Here's how the part is built. I have some questions about the finished solid (model axes, mm). Face numbers are marked on the shaded views. A direction names the side the tool comes from. Coordinates: 2 decimals unless noted, no trailing zeros. Write each loop counter-clockwise with the first axis right and the second up, starting at its lowest first coordinate (ties: lowest second). Pieces come first, ordered by that corner, then holes. Notation, with made-up numbers: (18.5, 41.5) -> (67.5, 41.5) arc R17 cw to (67.5, 73.5) -> close; hole circle Ø4 at (-31, -22). An arc over 180 degrees is marked (long way). Use CSV: the item, a comma, the result in double quotes. Start each with the question number.
```python
from build123d import *

# Parameters (mm, degrees)
SKETCH1_W           = 70
SKETCH1_H           = 170
SKETCH1_W_2         = 40
SKETCH1_H_2         = 140
BOSS_EXTRUDE1_DEPTH = 20


# Read off the part's stored shape, not the designer's step: Hole1
with BuildPart() as part:
    # Sketch1 → Boss-Extrude1 (new body)
    with BuildSketch(Plane(origin=(0, 0, 0), x_dir=(0, 0, -1), z_dir=(1, 0, 0))):
        Rectangle(SKETCH1_W, SKETCH1_H)
        Rectangle(SKETCH1_W_2, SKETCH1_H_2, mode=Mode.SUBTRACT)
    extrude(amount=BOSS_EXTRUDE1_DEPTH)

    # Hole1 outline → Hole1 (revolve, cut)
    with BuildSketch(Plane(origin=(10.287047222, -0.784426919, 0), x_dir=(1, 0, 0), z_dir=(0, -1, 0))):
        Polygon((0, 20), (2.555546136, 20), (2.031734593, 35), (0, 35), align=None)
        Polygon((3.952376915, -20), (0, -20), (0, -35), (4.476188458, -35), align=None)
    revolve(axis=Axis((10.287047222, -0.784426919, 0), (0, 0, 1)), mode=Mode.SUBTRACT)


solid = part.part
```
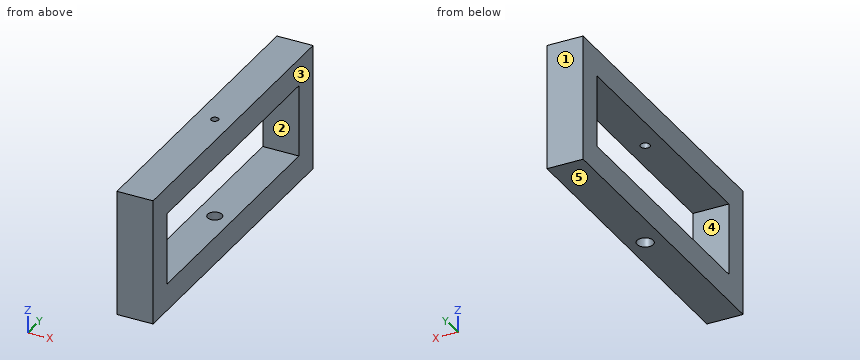
Item 1: If I drill on line 1 along Y through (x, z) = (16, 14); line 2 along Z through (x, y) = (7.5, 59.5); line 3 along Y through (x, z) = (10.75, -28), over which ranges is the centre line in solid material (lowest first)?
Item 2: Thinking about a two-plate mould opening in Y: for the marked faces 1, 2 and 3, which applies, +Y half, -Y half, draft (parallel to the pull), parting line (faces both ways), or undercut?
Item 3: I want a section at A-A on y = -26. Please give me the cut outline in (x, z).
Item 4: Which directions (+Z, -Z, +X, -X, +Y, -Y) give clear straight access to the entire face, cutting with the end or side of a thin tool? Please do the marked faces 4 and 5.
Item 5: I want a section at D-D on z = -30. Please give me the cut outline in (x, y), then the cut area to 3 significant figures.
Item 6: I want a section at B-B on z = -6.5. Please give me the cut outline in (x, y).
Item 7: I want a section at C-C on x = 17.5. Please give me the cut outline in (y, z).
Geometry says:
1,line 1,"-85 to -70, 70 to 85"
1,line 2,"-35 to -20, 20 to 35"
1,line 3,"-85 to -4.99, 3.42 to 85"
2,face 1,"+Y half"
2,face 2,"undercut"
2,face 3,"draft"
3,outline,"(0, -35) -> (20, -35) -> (20, -20) -> (0, -20) -> close; (0, 20) -> (20, 20) -> (20, 35) -> (0, 35) -> close"
4,face 4,"+X, -X"
4,face 5,"-Z, +X, -X, +Y, -Y"
5,outline,"(0, -85) -> (20, -85) -> (20, 85) -> (0, 85) -> close; hole circle Ø8.6 at (10.29, -0.78)"
5,area,"3,340 mm2"
6,outline,"(0, -85) -> (20, -85) -> (20, -70) -> (0, -70) -> close; (0, 70) -> (20, 70) -> (20, 85) -> (0, 85) -> close"
7,outline,"(-85, -35) -> (85, -35) -> (85, 35) -> (-85, 35) -> close; hole (-70, -20) -> (70, -20) -> (70, 20) -> (-70, 20) -> close"
